Part model, mm, in its own coordinate system. A direction names the side the tool comes from. Round coordinates to 2 decimals unless told otherwise and drop trailing zeros. Loops run counter-clockwise (first coordinate to the right, second up) from the corner with the lowest first, then second, coordinate; pieces in that order, holes last.
1) Mould opens along X. For faces 4 (the flat face through (-4, 14, -1)), 5 (the cylindrical face through (-2.44, -0.22, 8.62)), 6 (the cylindrical face through (0.47, 12.521, -11.445)) say: +X half, -X half, draft (parallel to the pull), parting line (faces both ways), or undercut.
2) Band-saw the part on C-C, the plane x = -0.5. Write the cut outline in (y, z).
3) Band-saw the part on D-D, the plane z = -5.75. Write the cut outline in (x, y).
4) Drop flat-ended pins along their axis: P1, Ø2.5, axis at y = -13, z = 3.5, coming from the +X side; P2, Ø3.5, axis at y = -13, z = 3.5, coming from the -X side; P3, Ø10, axis at y = 11, z = 7.5, coming from the -X side; P4, Ø9.5, axis at x = -5.5, y = -2, coming from the -Z side. Give the stop position or say it passes through.
5) Band-saw the part on A-A, the plane z = 3. Write the cut outline in (x, y), then the cut area to 3 significant figures.
6) Band-saw the part on B-B, the plane y = 1. Write the cut outline in (x, z), then the cut area to 3 significant figures.
7) Probe line 1 (Y direction, x = -7.25, z = -5); line 2 (Z direction, x = -0.25, y = -1.5); line 3 (X direction, y = 13, z = 4.25). List the from-to ranges inside material, lowest first.
8) 3-axis set-ups, long thin cutter, end or side, ignore diameter. For faces 1 (the flat face through (-10.026, -12, 0)), 2 (the flat face through (-4, 11, -3)), 3 (the flat face through (1.974, -12, 0)): which of +Z, -Z, +X, -X, +Y, -Y reach the whole face in a straight line?
from build123d import *

# Parameters (mm, degrees)
EXTRUDE_2_DEPTH     = 14
SKETCH_4_R          = 1.5
CUT_EXTRUDE_2_DEPTH = 21
EXTRUDE_3_DEPTH     = 14
SKETCH_5_W          = 12
SKETCH_5_H          = 26.808765345
CUT_EXTRUDE_3_DEPTH = 11
SKETCH_7_R          = 1
CUT_EXTRUDE_4_DEPTH = 11
SKETCH_8_R          = 2
CUT_EXTRUDE_5_DEPTH = 1
SKETCH_9_W          = 1
SKETCH_9_H          = 28
CUT_EXTRUDE_6_DEPTH = 10


with BuildPart() as part:
    # 草图1 → 凸台-拉伸2 (new body, symmetric)
    with BuildSketch(Plane(origin=(0, 0, 0), x_dir=(1, 0, 0), z_dir=(0, 1, 0))):
        with BuildLine():
            Line((-5.026135275, 12.870728162), (-3.026135275, 12.870728162))
            ThreePointArc((-3.026135275, 12.870728162), (0.50939863, 11.406262068), (1.973864725, 7.870728162))
            Line((1.973864725, 7.870728162), (1.973864725, -8.129271838))
            Line((1.973864725, -8.129271838), (-10.026135275, -8.129271838))
            Line((-10.026135275, -8.129271838), (-10.026135275, 7.870728162))
            ThreePointArc((-10.026135275, 7.870728162), (-8.561669181, 11.406262068), (-5.026135275, 12.870728162))
        make_face()
    extrude(amount=EXTRUDE_2_DEPTH, both=True)

    # 草图4 → 切除-拉伸2 (cut, symmetric)
    with BuildSketch(Plane(origin=(0, 0, 0), x_dir=(1, 0, 0), z_dir=(0, 1, 0))):
        with Locations((-4.026135275, 6.870728162)):
            Circle(SKETCH_4_R)
    extrude(amount=CUT_EXTRUDE_2_DEPTH, both=True, mode=Mode.SUBTRACT)

    # 草图2 → 凸台-拉伸3 (add, symmetric)
    with BuildSketch(Plane(origin=(0, 0, 0), x_dir=(1, 0, 0), z_dir=(0, 1, 0))):
        with BuildLine():
            Line((-10.026135275, -8.129271838), (1.973864725, -8.129271838))
            ThreePointArc((1.973864725, -8.129271838), (4.095185068, -9.007951494), (4.973864725, -11.129271838))
            Line((4.973864725, -11.129271838), (4.973864725, -12.129271838))
            Line((4.973864725, -12.129271838), (-13.026135275, -12.129271838))
            Line((-13.026135275, -12.129271838), (-13.026135275, -11.129271838))
            ThreePointArc((-13.026135275, -11.129271838), (-12.147455619, -9.007951494), (-10.026135275, -8.129271838))
        make_face()
    extrude(amount=EXTRUDE_3_DEPTH, both=True)

    # 草图5 → 切除-拉伸3 (cut, symmetric)
    with BuildSketch(Plane(origin=(0, 0, 0), x_dir=(1, 0, 0), z_dir=(0, 1, 0))):
        with Locations((-4.026135275, 5.275110834)):
            Rectangle(SKETCH_5_W, SKETCH_5_H)
    extrude(amount=CUT_EXTRUDE_3_DEPTH, both=True, mode=Mode.SUBTRACT)

    # 草图7 → 切除-拉伸4 (cut, symmetric)
    with BuildSketch(Plane.XY.offset(12.129271838)):
        with Locations((-4.026135275, 1)):
            Circle(SKETCH_7_R)
    extrude(amount=CUT_EXTRUDE_4_DEPTH, both=True, mode=Mode.SUBTRACT)

    # 草图8 → 切除-拉伸5 (cut)
    with BuildSketch(Plane(origin=(0, 0, 8.129271838), x_dir=(-1, 0, 0), z_dir=(0, 0, -1))):
        with Locations((4.026135275, 1)):
            Circle(SKETCH_8_R)
    extrude(amount=-CUT_EXTRUDE_5_DEPTH, mode=Mode.SUBTRACT)

    # 草图9 → 切除-拉伸6 (cut)
    with BuildSketch(Plane.XY.offset(12.129271838)):
        with Locations((-12.526135275, 0)):
            Rectangle(SKETCH_9_W, SKETCH_9_H)
        with Locations((4.473864725, 0)):
            Rectangle(SKETCH_9_W, SKETCH_9_H)
    extrude(amount=-CUT_EXTRUDE_6_DEPTH, mode=Mode.SUBTRACT)


solid = part.part
Reported:
1. face 4: draft
1. face 5: undercut
1. face 6: +X half
2. outline: (-14, -12.19) - (-11, -12.19) - (-11, 8.13) - (11, 8.13) - (11, -12.19) - (14, -12.19) - (14, 12.13) - (-14, 12.13) - close
3. outline: (-10.03, -14) - (-5.02, -14) - (-5.02, -11) - (-10.03, -11) - close; (-10.03, 11) - (-5.02, 11) - (-5.02, 14) - (-10.03, 14) - close; (-3.03, -14) - (1.97, -14) - (1.97, -11) - (-3.03, -11) - close; (-3.03, 11) - (1.97, 11) - (1.97, 14) - (-3.03, 14) - close
4. P1: stops at x = 1.97
4. P2: stops at x = -10.03
4. P3: stops at x = -12.03
4. P4: stops at z = 8.13
5. outline: (-10.03, -14) - (1.97, -14) - (1.97, -11) - (-10.03, -11) - close; (-10.03, 11) - (1.97, 11) - (1.97, 14) - (-10.03, 14) - close
5. area: 72.0 mm2
6. outline: (-12.03, 8.89) arc R3 ccw to (-10.03, 8.13) - (-6.03, 8.13) - (-6.03, 9.13) - (-5.03, 9.13) - (-5.03, 12.13) - (-12.03, 12.13) - close; (-3.03, 9.13) - (-2.03, 9.13) - (-2.03, 8.13) - (1.97, 8.13) arc R3 ccw to (3.97, 8.89) - (3.97, 12.13) - (-3.03, 12.13) - close
6. area: 53.0 mm2
7. line 1: y = -14 to -11, 11 to 14
7. line 2: z = 8.13 to 12.13
7. line 3: x = -10.03 to 1.97
8. face 1: -Z, -X, +Y, -Y
8. face 2: -Z, +X, -X
8. face 3: -Z, +X, +Y, -Y
